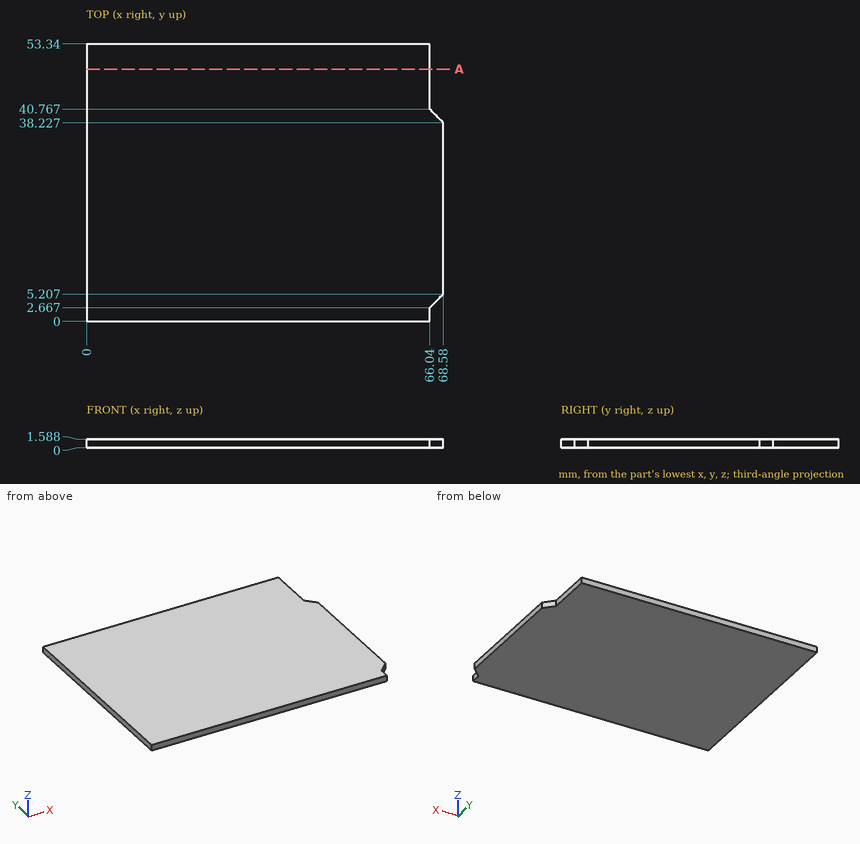
Geometry: see drawing. Coordinates: mm, zero at the bounding-box minimum. Round coordinates to 2 decimals unless told otherwise and drop trailing zeros. Loops run counter-clockwise (first coordinate to the right, second up) from the corner with the lowest first, then second, coordinate; pieces in that order, holes last.
(1) Section query A-A (y = 48.5). Output: boundary loops of the cut face in (x, z).
From the geometry:
outline: (0, 0) - (66.04, 0) - (66.04, 1.59) - (0, 1.59) - close
(2) Material intervals for probe 1 along X at (y, z) = (51, 0.95); probe 2 along X at (y, z) = (4, 0.3), sorted ascending.
From the geometry:
probe 1: x = 0 to 66.04
probe 2: x = 0 to 67.37
(3) Contact query for flat-ended pins moving along their axis: pin 1 Ø0.8 at (y, z) = (49.5, 0.5) entering from +X; pin 2 Ø6 at (x, y) = (18, 6.5) entering from -Z. Output: stop coordinate, or through.
From the geometry:
pin 1: stops at x = 66.04
pin 2: stops at z = 0
